```python
from build123d import *

# Parameters (mm, degrees)
EXTRUDE_2_DEPTH     = 25
EXTRUDE_3_DEPTH     = 45
SKETCH_2_R          = 31.5
EXTRUDE_4_DEPTH     = 30
SKETCH_3_W          = 30
SKETCH_3_H          = 172.84779514
CUT_EXTRUDE_1_DEPTH = 15


with BuildPart() as part:
    # Sketch 1 → Extrude 2 (new body)
    with BuildSketch(Plane(origin=(0, 0, 0), x_dir=(1, 0, 0), z_dir=(0, 1, 0))):
        with BuildLine():
            ThreePointArc((0, -85), (-85, 0), (0, 85))
            Line((0, 85), (171, 85))
            Line((171, 85), (171, 115))
            Line((171, 115), (0, 115))
            ThreePointArc((0, 115), (-115, 0), (0, -115))
            Line((0, -115), (171, -115))
            Line((171, -115), (171, -85))
            Line((171, -85), (0, -85))
        make_face()
        with BuildLine():
            Line((171, 85), (0, 85))
            ThreePointArc((0, 85), (-85, 0), (0, -85))
            Line((0, -85), (171, -85))
            Line((171, -85), (171, -75))
            Line((171, -75), (0, -75))
            ThreePointArc((0, -75), (-75, 0), (0, 75))
            Line((0, 75), (171, 75))
            Line((171, 75), (171, 85))
        make_face()
    extrude(amount=EXTRUDE_2_DEPTH)

    # Sketch 1_5 → Extrude 3 (add)
    with BuildSketch(Plane(origin=(0, 0, 0), x_dir=(1, 0, 0), z_dir=(0, 1, 0))):
        with BuildLine():
            ThreePointArc((0, -85), (-85, 0), (0, 85))
            Line((0, 85), (171, 85))
            Line((171, 85), (171, 115))
            Line((171, 115), (0, 115))
            ThreePointArc((0, 115), (-115, 0), (0, -115))
            Line((0, -115), (171, -115))
            Line((171, -115), (171, -85))
            Line((171, -85), (0, -85))
        make_face()
    extrude(amount=EXTRUDE_3_DEPTH)

    # Sketch 2 → Extrude 4 (add)
    with BuildSketch(Plane.XY.offset(-85)):
        with BuildLine():
            Line((171, 25), (53, 25))
            Line((53, 25), (53, 104))
            ThreePointArc((53, 104), (112, 163), (171, 104))
            Line((171, 104), (171, 25))
        make_face()
        with Locations((112, 104)):
            Circle(SKETCH_2_R, mode=Mode.SUBTRACT)
    extrude_4 = extrude(amount=-EXTRUDE_4_DEPTH)

    # Sketch 3 → Cut-Extrude 1 (cut)
    with BuildSketch(Plane(origin=(0, 0, -115), x_dir=(-1, 0, 0), z_dir=(0, 0, -1))):
        with Locations((-112, 0)):
            Rectangle(SKETCH_3_W, SKETCH_3_H)
    cut_extrude_1 = extrude(amount=-CUT_EXTRUDE_1_DEPTH, mode=Mode.SUBTRACT)

    # Mirror 4: Extrude 4, Cut-Extrude 1 across plane
    add(extrude_4.mirror(Plane.XY))
    add(cut_extrude_1.mirror(Plane.XY), mode=Mode.SUBTRACT)


solid = part.part
```
Check sheet for the modelled part. Datum: model origin and axes. Units: mm. A direction names the side the tool comes from. Round coordinates to 2 decimals unless told otherwise and drop trailing zeros. Order: outer loops, then holes, each group sorted by start corner. A loop starts at its lowest first (then second) coordinate and runs counter-clockwise, first axis right, second up.
1) Mould release check, pull along Z, two halves, no side actions. Record for faces 4 (the flat face through (112, 39, 100)), 5 (the cylindrical face through (110.703, 162.986, 99.79)), 6 (the flat face through (87, 12, 75)): +Z half, -Z half, draft (parallel to the pull), parting line (faces both ways), or undercut.
2) Go/stop test with flat-tipped pins: pin 1 Ø4.5 at (y, z) = (48.5, 105) entering from -X; pin 2 Ø12 at (x, y) = (-56.5, 31.5) entering from -Z; pin 3 Ø10 at (y, z) = (16.5, 67) entering from -X; pin 4 Ø10 at (x, z) = (20, -72) entering from -Y. Record where each tip stops, or that it passes through.
3) Section check B-B (y = 59.5). Record the boundary of the cut face in (x, z).
4) Tool access check on faces 1 (the flat face through (112, 39, -100)), 2 (the flat face through (103, 62, -85)), 3 (the flat face through (97, 38, 108)). Record the directions out of +Z, -Z, +X, -X, +Y, -Y that give a thin tool (end or side, any length) a straight path to the whole face; none if there is none.
5) Section check A-A (x = 112). Record the boundary of the cut face in (y, z), and give its area (4 significant figures).
6) Section check D-D (y = 40.5). Record the boundary of the cut face in (x, z), and give its area (3 significant figures).
7) Scan lines: line 1 (Z direction, x = 149, y = 98.5); line 2 (Z direction, x = 109, y = 62.5); line 3 (X direction, y = 104, z = -94.75). Record each from-to range of solid material in increasing order.
8) Section check C-C (x = 43.5). Record the boundary of the cut face in (y, z), and give its area (3 significant figures).
Result:
1. face 4: +Z half
1. face 5: draft
1. face 6: undercut
2. pin 1: stops at x = 53
2. pin 2: stops at z = -103.32
2. pin 3: stops at x = -96.86
2. pin 4: stops at y = 0
3. outline: (53, -115) - (97, -115) - (97, -100) - (127, -100) - (127, -115) - (171, -115) - (171, -85) - (53, -85) - close; (53, 85) - (171, 85) - (171, 115) - (127, 115) - (127, 100) - (97, 100) - (97, 115) - (53, 115) - close
4. face 1: -Z, -Y
4. face 2: +X, +Y
4. face 3: +Z, -Y
5. outline: (0, -100) - (72.5, -100) - (72.5, -85) - (25, -85) - (25, -75) - (0, -75) - close; (0, 75) - (25, 75) - (25, 85) - (72.5, 85) - (72.5, 100) - (0, 100) - close; (135.5, -115) - (163, -115) - (163, -85) - (135.5, -85) - close; (135.5, 85) - (163, 85) - (163, 115) - (135.5, 115) - close
5. area: 4,325 mm2
6. outline: (0, -115) - (97, -115) - (97, -100) - (127, -100) - (127, -115) - (171, -115) - (171, -85) - (0, -85) arc R85 cw to (0, 85) - (171, 85) - (171, 115) - (127, 115) - (127, 100) - (97, 100) - (97, 115) - (0, 115) arc R115 ccw to start
6. area: 18,800 mm2
7. line 1: z = -115 to -85, 85 to 115
7. line 2: z = -100 to -85, 85 to 100
7. line 3: x = 53 to 80.5, 143.5 to 171
8. outline: (0, -115) - (45, -115) - (45, -85) - (25, -85) - (25, -75) - (0, -75) - close; (0, 75) - (25, 75) - (25, 85) - (45, 85) - (45, 115) - (0, 115) - close
8. area: 3,200 mm2
